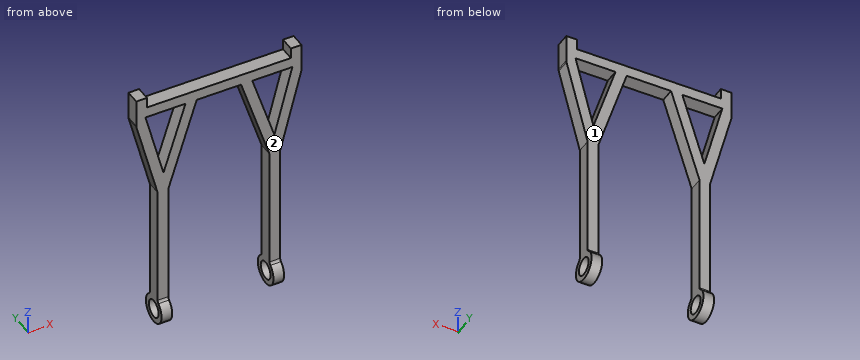
```python
from build123d import *

# Parameters (mm, degrees)
BOSS_EXTRUDE1_DEPTH     = 1
BOSS_EXTRUDE2_START     = 7.125
BOSS_EXTRUDE2_DEPTH     = 1.5
BOSS_EXTRUDE3_START     = -8.625
BOSS_EXTRUDE3_DEPTH     = 1.5
SKETCH3_R               = 1.25
CUT_EXTRUDE1_DEPTH      = 12.625
CUT_EXTRUDE1_DEPTH_BACK = 12.625


with BuildPart() as part:
    # Sketch1 → Boss-Extrude1 (new body, symmetric)
    with BuildSketch(Plane(origin=(0, 0, 0), x_dir=(1, 0, 0), z_dir=(0, 1, 0))):
        with BuildLine():
            Line((-10.125, -0.75), (0, -0.75))
            Line((0, -0.75), (0, 0.75))
            Line((0, 0.75), (-3.125, 0.75))
            Line((-3.125, 0.75), (-7.125, 13.25))
            Line((-7.125, 13.25), (-7.125, 30.25))
            Line((-7.125, 30.25), (-8.625, 30.25))
            Line((-8.625, 30.25), (-8.625, 13.25))
            Line((-8.625, 13.25), (-11.592617272, 1.874133789))
            ThreePointArc((-11.592617272, 1.874133789), (-11.61687128, 1.748957182), (-11.625, 1.621711892))
            Line((-11.625, 1.621711892), (-11.625, -0.75))
            Line((-11.625, -0.75), (-11.625, -2.25))
            Line((-11.625, -2.25), (-10.125, -2.25))
            Line((-10.125, -2.25), (-10.125, -0.75))
        make_face()
        Polygon((-4.69992857, 0.75), (-7.804648328, 10.452249246), (-10.335669871, 0.75), align=None, mode=Mode.SUBTRACT)
    boss_extrude1 = extrude(amount=BOSS_EXTRUDE1_DEPTH, both=True)

    # Mirror1: Boss-Extrude1 across plane
    add(boss_extrude1.mirror(Plane(origin=(0, 0, 0), x_dir=(0, 0, 1), z_dir=(1, 0, 0))))

    # Sketch2 → Boss-Extrude2 (add)
    with BuildSketch(Plane(origin=(0, 0, 0), x_dir=(0, 0, -1), z_dir=(1, 0, 0)).offset(BOSS_EXTRUDE2_START)):
        with BuildLine():
            Line((30.25, 1), (30.25, -1))
            ThreePointArc((30.25, -1), (30.473606798, -1.052786405), (30.65, -1.2))
            ThreePointArc((30.65, -1.2), (34.25, 0), (30.65, 1.2))
            ThreePointArc((30.65, 1.2), (30.473606798, 1.052786405), (30.25, 1))
        make_face()
    extrude(amount=BOSS_EXTRUDE2_DEPTH)

    # Sketch2<2> → Boss-Extrude3 (add)
    with BuildSketch(Plane(origin=(0, 0, 0), x_dir=(0, 0, -1), z_dir=(1, 0, 0)).offset(BOSS_EXTRUDE3_START)):
        with BuildLine():
            Line((30.25, 1), (30.25, -1))
            ThreePointArc((30.25, -1), (30.473606798, -1.052786405), (30.65, -1.2))
            ThreePointArc((30.65, -1.2), (34.25, 0), (30.65, 1.2))
            ThreePointArc((30.65, 1.2), (30.473606798, 1.052786405), (30.25, 1))
        make_face()
    extrude(amount=BOSS_EXTRUDE3_DEPTH)

    # Sketch3 → Cut-Extrude1 (cut, two sides)
    with BuildSketch(Plane(origin=(0, 0, 0), x_dir=(0, 0, -1), z_dir=(1, 0, 0))) as cut_extrude1_sk:
        with Locations((32.25, 0)):
            Circle(SKETCH3_R)
    extrude(amount=CUT_EXTRUDE1_DEPTH, mode=Mode.SUBTRACT)
    extrude(cut_extrude1_sk.sketch, amount=-CUT_EXTRUDE1_DEPTH_BACK, mode=Mode.SUBTRACT)


solid = part.part
```
Check sheet for the modelled part. Datum: model origin and axes. Units: mm. Face numbers are marked on the shaded views. A direction names the side the tool comes from. Round coordinates to 2 decimals unless told otherwise and drop trailing zeros. Write each loop counter-clockwise with the first axis right and the second up, starting at its lowest first coordinate (ties: lowest second). Pieces come first, ordered by that corner, then holes. Notation, with made-up numbers: (85, 16.5) -> (92, 16.5) arc R20 cw to (92, 47.5) -> close; hole circle Ø2 at (-17, -32.75). An arc over 180 degrees is marked (long way). One line per question, with ' | ' between items. Start each with the question number.
1. Scan lines: line 1 along X through (y, z) = (0.9, -15) (3 decimals); line 2 along Y through (x, z) = (8.2, -32.25); line 3 along X through (y, z) = (0.4, -5) (3 decimals). Record each from-to range of solid material in increasing order. Write a range as from..to.
2. Sectioned sample at C-C, the plane x = -8.25. Record the cut outline in (y, z), then the cut area to 3 significant figures.
3. Depth check by flat-ended pin: pin 1 (2 mm diameter, centred on y = -1, z = -27.5, fed in from +X) (3 decimals); pin 2 (1 mm diameter, centred on y = 0, z = -20, fed in from -X) (3 decimals); pin 3 (2 mm diameter, centred on x = -0.5, y = 0, fed in from -Z). Enter the tip coordinate at first touch or a pass-through.
4. Set-up check for the marked faces 1 and 2: record each of +Z, -Z, +X, -X, +Y, -Y from which the full face is reachable in a straight line by a thin tool's end or side.
5. Sectioned sample at A-A, the plane y = 0. Count the separate pieces of the cut face and the enclosed holes in it, then the cut area to 3 significant figures.
6. Sectioned sample at D-D, the plane z = -32.25. Record the cut outline in (x, y) (3 decimals), then the cut area to 3 significant figures.
7. Sectioned sample at B-B, the plane z = -14.5. Record the cut outline in (x, y) (3 decimals), then the cut area to 3 significant figures.
Taken from the geometry:
1) line 1: x = -8.625..-7.125, 7.125..8.625 | line 2: y = -2..-1.25, 1.25..2 | line 3: x = -10.777..-9.227, -6.06..-4.485, 4.485..6.06, 9.227..10.777
2) outline: (-1.2, -30.65) arc R2 ccw (long way) to (1.2, -30.65) arc R0.5 cw to (1, -30.25) -> (1, -8.75) -> (-1, -8.75) -> (-1, -30.25) arc R0.5 cw to start; (-1, -0.75) -> (1, -0.75) -> (1, 0.75) -> (-1, 0.75) -> close; hole circle Ø2.5 at (0, -32.25) | area: 53.9 mm^2
3) pin 1: stops at x = 8.625 | pin 2: stops at x = -8.625 | pin 3: stops at z = -0.75
4) face 1: +Z, +X, -X, +Y | face 2: +Z, +X, -X, -Y
5) separate pieces: 3 | enclosed holes: 2 | area: 168 mm^2
6) outline: (-8.625, -2) -> (-7.125, -2) -> (-7.125, -1.25) -> (-8.625, -1.25) -> close; (-8.625, 1.25) -> (-7.125, 1.25) -> (-7.125, 2) -> (-8.625, 2) -> close; (7.125, -2) -> (8.625, -2) -> (8.625, -1.25) -> (7.125, -1.25) -> close; (7.125, 1.25) -> (8.625, 1.25) -> (8.625, 2) -> (7.125, 2) -> close | area: 4.50 mm^2
7) outline: (-8.625, -1) -> (-7.125, -1) -> (-7.125, 1) -> (-8.625, 1) -> close; (7.125, -1) -> (8.625, -1) -> (8.625, 1) -> (7.125, 1) -> close | area: 6.00 mm^2
